```python
from build123d import *

# Parameters (mm, degrees)
F1_DEPTH = 25.4


with BuildPart() as f1:
    # F0 (on Front) → F1 (new body)
    with BuildSketch(Plane.XZ):
        Polygon((-25.515185, 49.338989), (-82.486942, 49.338989), (-110.97282, 0), (-82.486942, -49.338989), (-25.515185, -49.338989), (2.970694, 0), align=None)
        Polygon((60.591042, 19.869066), (-25.515185, 49.338989), (2.970694, 0), (-25.515185, -49.338989), (60.591042, -19.869066), (43.383926, -9.934533), (43.383926, 9.934533), align=None)
        Polygon((77.798158, 9.934533), (60.591042, 19.869066), (43.383926, 9.934533), (43.383926, -9.934533), (60.591042, -19.869066), (77.798158, -9.934533), align=None)
    extrude(amount=F1_DEPTH)


solid = f1.part
```
The model under review builds one solid part; all positions refer to its coordinate system, in mm. Give positions to 0.01 mm unless a question says otherwise; leave off trailing zeros. Write each loop counter-clockwise with the first axis right and the second up, starting at its lowest first coordinate (ties: lowest second). Pieces come first, ordered by that corner, then holes. Notation, with made-up numbers: (-32, 52.5) -> (12, 52.5) arc R22 cw to (12, 83.5) -> close; hole circle Ø6 at (-4, 85.5). An arc over 180 degrees is marked (long way). Put each result on its own line as item: value.
(1) We need section A-A, the plane y = -16. Give the boundary of the cut face in (x, z), and give its area (3 significant figures).
Results are:
outline: (-110.97, 0) -> (-82.49, -49.34) -> (-25.52, -49.34) -> (60.59, -19.87) -> (77.8, -9.93) -> (77.8, 9.93) -> (60.59, 19.87) -> (-25.52, 49.34) -> (-82.49, 49.34) -> close
area: 13,500 mm²
(2) We need section C-C, the plane x = 15. Give the boundary of the cut face in (y, z), and give its area (3 significant figures).
Results are:
outline: (-25.4, -35.47) -> (0, -35.47) -> (0, 35.47) -> (-25.4, 35.47) -> close
area: 1,800 mm²
(3) We need section B-B, the plane z = 39.5. Give the boundary of the cut face in (x, y), and give its area (3 significant figures).
Results are:
outline: (-88.17, -25.4) -> (3.23, -25.4) -> (3.23, 0) -> (-88.17, 0) -> close
area: 2,320 mm²
(4) To check wall thickness, follow probe 1 along X at (y, z) = (-4, -8); probe 2 along Z at (x, y) = (-97.5, -15.5); probe 3 along Z at (x, y) = (-12, -19.5). State the ranges of each line that lie inside material, in increasing order. Write a range as from..to.
Results are:
probe 1: -106.35..77.8
probe 2: -23.34..23.34
probe 3: -44.71..44.71
(5) For pin 1 Ø6 at (x, y) = (-88.5, -18.5) entering from -Z; pin 2 Ø5 at (x, z) = (2, 21.5) entering from +Y; pin 3 Ø8 at (y, z) = (-20.5, 14) entering from -X; pin 4 Ø8 at (y, z) = (-7, 20.5) entering from -X, all flat-tipped, find the tip position at first contact; note any pin that passes through.
Results are:
pin 1: z = -44.12
pin 2: y = 0
pin 3: x = -105.2
pin 4: x = -101.45
